Check sheet for the drawn part. Datum: minimum x, y, z corner. Units: mm. Give positions to 0.01 mm unless a question says otherwise; leave off trailing zeros. Loops run counter-clockwise (first coordinate to the right, second up) from the corner with the lowest first, then second, coordinate; pieces in that order, holes last. Notation, with made-up numbers: (-40, 26.5) -> (10, 26.5) arc R23 ccw to (10, 57.5) -> close; hole circle Ø10 at (22.5, 5.5). An arc over 180 degrees is marked (long way). One line per question, with ' | ' between items.
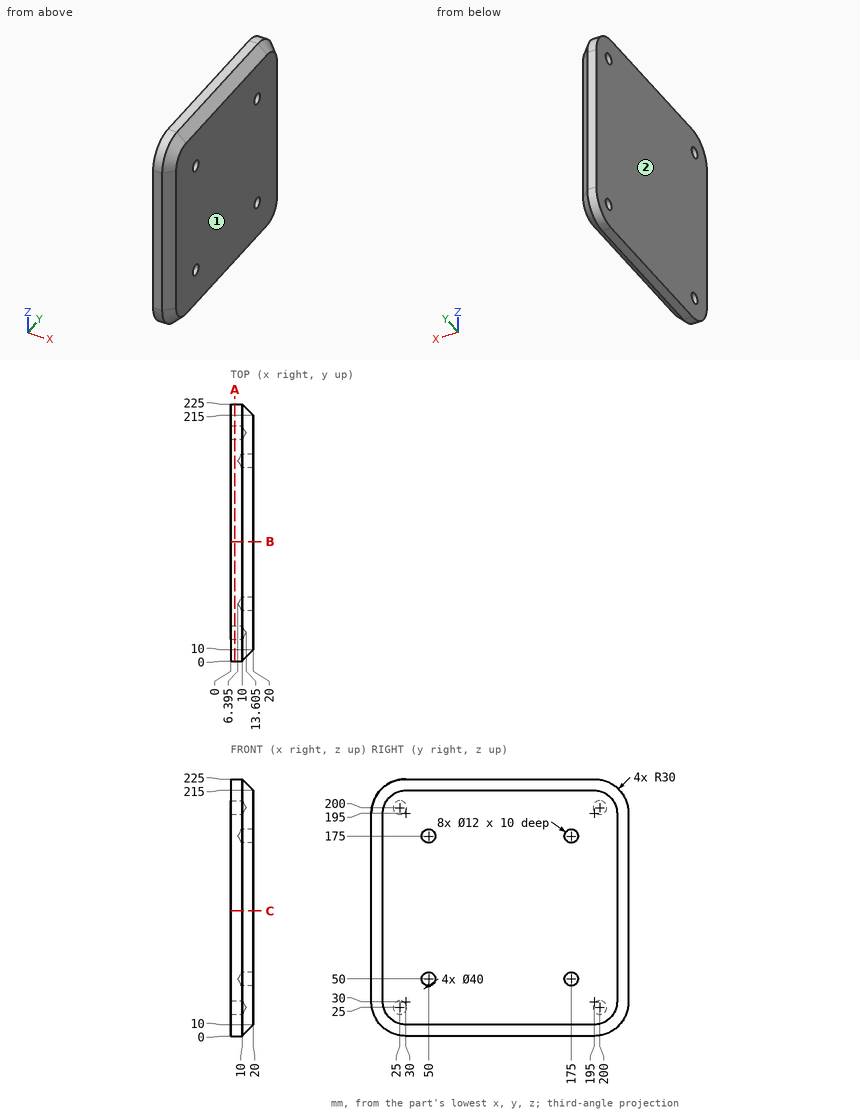
Item 1: Scan lines: probe 1 along Z at (x, y) = (13, 50); probe 2 along Y at (x, z) = (8, 199); probe 3 along Z at (x, y) = (14.25, 50). Record each from-to range of solid material in increasing order.
Result:
probe 1: 3 to 44, 56 to 169, 181 to 222 | probe 2: 0.27 to 19.08, 30.92 to 194.08, 205.92 to 224.73 | probe 3: 4.25 to 44, 56 to 169, 181 to 220.75
Item 2: Depth check by flat-ended pin: pin 1 Ø9.5 at (y, z) = (25, 200) entering from -X. Enter the tip coordinate at first touch or a pass-through.
Result:
pin 1: x = 10.75
Item 3: Release check for a two-part mould opening along X. For the marked faces 1 and 2 record: pulls with the +X half, pulls with the -X half, needs draft (parallel to the pull), parting line crosses it, or undercut.
Result:
face 1: pulls with the +X half | face 2: pulls with the -X half
Item 4: Sectioned sample at B-B (y = 104.5). Record the cut outline in (x, z), plus the area to 3 significant figures.
Result:
outline: (0, 0) -> (10, 0) -> (20, 10) -> (20, 215) -> (10, 225) -> (0, 225) -> close | area: 4,400 mm2
Item 5: Sectioned sample at A-A (x = 3.75). Record the cut outline in (y, z).
Result:
outline: (0, 30) arc R30 ccw to (30, 0) -> (195, 0) arc R30 ccw to (225, 30) -> (225, 195) arc R30 ccw to (195, 225) -> (30, 225) arc R30 ccw to (0, 195) -> close; hole circle Ø12 at (25, 25); hole circle Ø12 at (25, 200); hole circle Ø12 at (200, 25); hole circle Ø12 at (200, 200)
